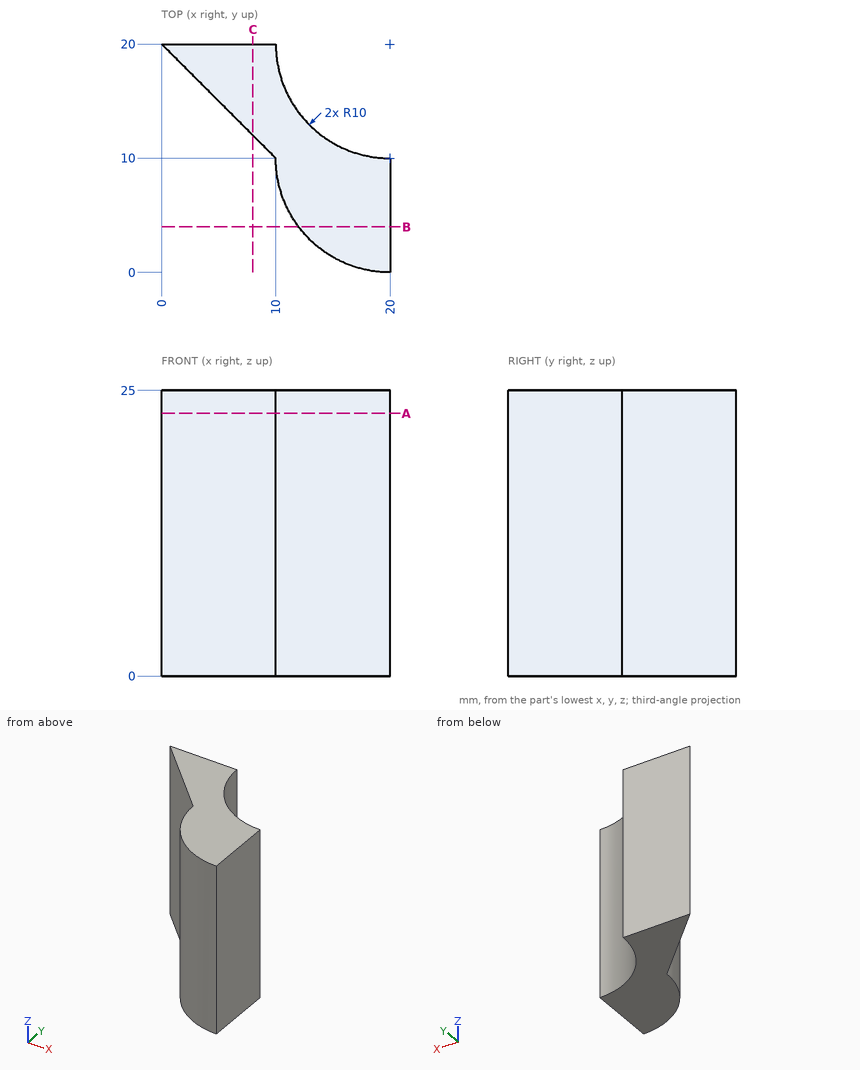
Geometry: see drawing. Coordinates: mm, zero at the bounding-box minimum. Coordinates: 2 decimals unless noted, no trailing zeros. Order: outer loops, then holes, each group sorted by start corner. A loop starts at its lowest first (then second) coordinate and runs counter-clockwise, first axis right, second up. Notation, with made-up numbers: M -22.75,-9.75 L 14.25,-9.75 A18 ccw 14.25,2.25 Z; hole C 32.5,21 d1. An arc over 180 degrees is marked long. Write item = value, one per line. Start each with the question number.
(1) First-contact query: P1, Ø4, axis at y = 4.5, z = 10.5, coming from the -X side; P2, Ø1.5, axis at y = 5.5, z = 4, coming from the -X side; P3, Ø4, axis at y = 18, z = 13.5, coming from the +X side. Flat tips, straight axial feed; report the tip coordinate or a pass-through.
(2) Section B-B on y = 4. Output: boundary loops of the cut face in (x, z).
(3) Line query: line 1 along Y through (x, z) = (3.25, 15.25); line 2 along Y through (x, z) = (13, 13); line 3 along X through (y, z) = (9.5, 13). Output: solid intervals per line, ascending. Write a range as [from, to].
(4) Section A-A on z = 23. Output: boundary loops of the cut face in (x, y), and give its area (3 significant figures).
Result set:
q1.P1 = 10.63
q1.P2 = 10.73
q1.P3 = 10.83
q2.outline = M 12,0 L 20,0 L 20,25 L 12,25 Z
q3.line_1 = [16.75, 20]
q3.line_2 = [2.86, 12.86]
q3.line_3 = [10.01, 20]
q4.outline = M 0,20 L 10,10 A10 ccw 20,0 L 20,10 A10 cw 10,20 Z
q4.area = 150 mm²
